Part model, mm, in its own coordinate system. Face numbers are marked on the shaded views. A direction names the side the tool comes from. Round coordinates to 2 decimals unless told otherwise and drop trailing zeros. Order: outer loops, then holes, each group sorted by start corner. A loop starts at its lowest first (then second) coordinate and runs counter-clockwise, first axis right, second up. Notation, with made-up numbers: (49, 65.5) - (106, 65.5) arc R20 cw to (106, 75.5) - close; hole circle Ø2 at (-6, 43.5). An arc over 180 degrees is marked (long way). Answer as a JSON object with one key per item and string values.
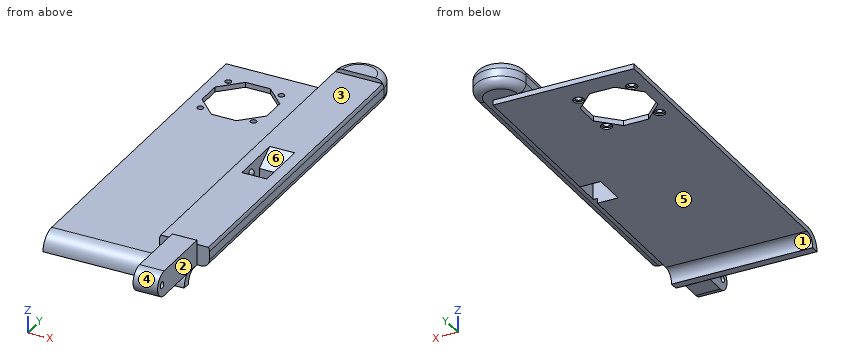
```python
from build123d import *

# Parameters (mm, degrees)
BOSS_EXTRUDE1_DEPTH = 7.5
FILLET1_R           = 5
SKETCH2_W           = 15
SKETCH2_H           = 20
CUT_EXTRUDE1_DEPTH  = 152.492574075
FILLET6_R           = 5
CUT_EXTRUDE2_DEPTH  = 152.848641746
BOSS_EXTRUDE2_DEPTH = 80
BOSS_EXTRUDE3_START = 5
BOSS_EXTRUDE3_DEPTH = 5
SKETCH12_W          = 12.5
SKETCH12_H          = 20
CUT_EXTRUDE3_DEPTH  = 3
SKETCH13_W          = 2.5
SKETCH13_H          = 200
CUT_EXTRUDE4_DEPTH  = 160.863222787
SKETCH14_R          = 1.85
CUT_EXTRUDE5_DEPTH  = 10
SKETCH15_R          = 3.25
CUT_EXTRUDE6_DEPTH  = 1
CUT_EXTRUDE7_DEPTH  = 7.5


with BuildPart() as part:
    # Sketch1 → Boss-Extrude1 (new, symmetric)
    with BuildSketch(Plane.XY):
        with BuildLine():
            Line((-15, 100), (-15, -100))
            Line((-15, -100), (-7.4, -100))
            Line((-7.4, -100), (-7.4, -150))
            Line((-7.4, -150), (7.4, -150))
            Line((7.4, -150), (7.4, -100))
            Line((7.4, -100), (15, -100))
            Line((15, -100), (15, 100))
            ThreePointArc((15, 100), (0, 115), (-15, 100))
        make_face()
    extrude(amount=BOSS_EXTRUDE1_DEPTH, both=True)

    # Fillet1
    fillet1_edges = [part.edges().sort_by_distance(p)[0] for p in [
        (-15, 0, -7.5),
        (0, 115, -7.5),
        (15, 0, 7.5),
        (0, 115, 7.5),
        (15, 0, -7.5),
        (-15, 0, 7.5),
    ]]
    fillet(fillet1_edges, radius=FILLET1_R)

    # Sketch2 → Cut-Extrude1 (cut, through all)
    with BuildSketch(Plane.XY.offset(7.5)):
        with Locations((0, -10)):
            Rectangle(SKETCH2_W, SKETCH2_H)
    extrude(amount=-CUT_EXTRUDE1_DEPTH, mode=Mode.SUBTRACT)

    # Sketch5 → Cut-Revolve1 (revolve, cut)
    with BuildSketch(Plane.XY):
        with BuildLine():
            Line((-7.4, -140), (-5.4, -140))
            ThreePointArc((-5.4, -140), (-5.985786438, -138.585786438), (-7.4, -138))
            Line((-7.4, -138), (-7.4, -140))
        make_face()
        with BuildLine():
            Line((7.4, -140), (5.4, -140))
            ThreePointArc((5.4, -140), (5.985786438, -138.585786438), (7.4, -138))
            Line((7.4, -138), (7.4, -140))
        make_face()
    revolve(axis=Axis((-35.580304025, -140, 0), (1, 0, 0)), mode=Mode.SUBTRACT)

    # Fillet6
    fillet6_edges = [part.edges().sort_by_distance(p)[0] for p in [
        (7.4, -150, 0),
        (-7.4, -150, 0),
    ]]
    fillet(fillet6_edges, radius=FILLET6_R)

    # Sketch7 → Cut-Extrude2 (cut, through all)
    with BuildSketch(Plane(origin=(7.4, 0, 0), x_dir=(0, 0, -1), z_dir=(1, 0, 0))):
        with BuildLine():
            Line((-7.5, -137.5), (-7.5, -150))
            Line((-7.5, -150), (7.5, -150))
            Line((7.5, -150), (7.5, -137.5))
            ThreePointArc((7.5, -137.5), (0, -145), (-7.5, -137.5))
        make_face()
    extrude(amount=-CUT_EXTRUDE2_DEPTH, mode=Mode.SUBTRACT)

    # Sketch9 → Revolve2 (revolve)
    with BuildSketch(Plane.XY):
        with BuildLine():
            Line((-7.5, -10), (-5.5, -10))
            ThreePointArc((-5.5, -10), (-6.085786438, -8.585786438), (-7.5, -8))
            Line((-7.5, -8), (-7.5, -10))
        make_face()
        with BuildLine():
            Line((7.5, -10), (5.5, -10))
            ThreePointArc((5.5, -10), (6.085786438, -8.585786438), (7.5, -8))
            Line((7.5, -8), (7.5, -10))
        make_face()
    revolve(axis=Axis((-32.251262552, -10, 0), (1, 0, 0)))

    # Sketch10 → Boss-Extrude2 (add)
    with BuildSketch(Plane(origin=(0, 0, 0), x_dir=(0, 0, -1), z_dir=(1, 0, 0))):
        with BuildLine():
            Line((7.5, -100), (7.5, 100))
            Line((7.5, 100), (10.5, 100))
            Line((10.5, 100), (10.5, -98.519259302))
            ThreePointArc((10.5, -98.519259302), (12.584119567, -103.288955309), (17.5, -105))
            Line((17.5, -105), (17.5, -110))
            ThreePointArc((17.5, -110), (10.428932188, -107.071067812), (7.5, -100))
        make_face()
    extrude(amount=-BOSS_EXTRUDE2_DEPTH)

    # Sketch11 → Boss-Extrude3 (add)
    with BuildSketch(Plane(origin=(0, 0, 0), x_dir=(0, 0, -1), z_dir=(1, 0, 0)).offset(BOSS_EXTRUDE3_START)):
        with BuildLine():
            Line((17.5, -110), (17.5, -105))
            ThreePointArc((17.5, -105), (12.584119567, -103.288955309), (10.5, -98.519259302))
            Line((10.5, -98.519259302), (10.5, 100))
            Line((10.5, 100), (7.5, 100))
            Line((7.5, 100), (7.5, -100))
            ThreePointArc((7.5, -100), (10.428932188, -107.071067812), (17.5, -110))
        make_face()
    extrude(amount=-BOSS_EXTRUDE3_DEPTH)

    # Sketch12 → Cut-Extrude3 (cut)
    with BuildSketch(Plane(origin=(0, 0, -10.5), x_dir=(-1, 0, 0), z_dir=(0, 0, -1))):
        with Locations((1.25, -10)):
            Rectangle(SKETCH12_W, SKETCH12_H)
    extrude(amount=-CUT_EXTRUDE3_DEPTH, mode=Mode.SUBTRACT)

    # Sketch13 → Cut-Extrude4 (cut, through all)
    with BuildSketch(Plane.ZY.offset(15)):
        with Locations((6.25, 0)):
            Rectangle(SKETCH13_W, SKETCH13_H)
    extrude(amount=-CUT_EXTRUDE4_DEPTH, mode=Mode.SUBTRACT)

    # Sketch14 → Cut-Extrude5 (cut)
    with BuildSketch(Plane(origin=(0, 0, -10.5), x_dir=(-1, 0, 0), z_dir=(0, 0, -1))):
        with Locations(Location((70, 51.480740698, 0), (0, 0, 90))):
            Circle(SKETCH14_R)
        with Locations(Location((70, 83.480740698, 0), (0, 0, 90))):
            Circle(SKETCH14_R)
        with Locations(Location((38, 83.480740698, 0), (0, 0, 90))):
            Circle(SKETCH14_R)
        with Locations(Location((38, 51.480740698, 0), (0, 0, 90))):
            Circle(SKETCH14_R)
        Polygon((61.5, 86.980740698), (46.5, 86.980740698), (34.5, 74.980740698), (34.5, 59.980740698), (46.5, 47.980740698), (61.5, 47.980740698), (73.5, 59.980740698), (73.5, 74.980740698), align=None)
    extrude(amount=-CUT_EXTRUDE5_DEPTH, mode=Mode.SUBTRACT)

    # Sketch15 → Cut-Extrude6 (cut)
    with BuildSketch(Plane(origin=(0, 0, -10.5), x_dir=(-1, 0, 0), z_dir=(0, 0, -1))):
        with Locations(Location((70, 83.480740698, 0), (0, 0, 90))):
            Circle(SKETCH15_R)
        with Locations(Location((38, 83.480740698, 0), (0, 0, 90))):
            Circle(SKETCH15_R)
        with Locations(Location((38, 51.480740698, 0), (0, 0, 90))):
            Circle(SKETCH15_R)
        with Locations(Location((70, 51.480740698, 0), (0, 0, 90))):
            Circle(SKETCH15_R)
    extrude(amount=-CUT_EXTRUDE6_DEPTH, mode=Mode.SUBTRACT)

    # Sketch16 → Cut-Extrude7 (cut, symmetric)
    with BuildSketch(Plane(origin=(0, 0, 0), x_dir=(0, 0, -1), z_dir=(1, 0, 0))):
        Polygon((2.5, 0), (-5, 12), (-5, 0), align=None)
    extrude(amount=CUT_EXTRUDE7_DEPTH, both=True, mode=Mode.SUBTRACT)


solid = part.part
```
Item 1: Tool access for the marked faces 4, 5 and 6: list every direction of +Z, -Z, +X, -X, +Y, -Y with a clear straight run to the whole face (end or side of a thin tool).
Taken from the geometry:
{"face 4": "+X, -X, -Y", "face 5": "-Z, +X, -X, +Y", "face 6": "+Z"}
Item 2: Drop flat-ended pins along their axis: P1, Ø6, axis at x = -38, y = 83.48, coming from the -Z side; P2, Ø3.5, axis at x = -50.5, z = -9.5, coming from the +Y side; P3, Ø1.5, axis at y = 33.5, z = -9.5, coming from the +X side. Give the stop position or say it passes through.
Taken from the geometry:
{"P1": "z = -9.5", "P2": "y = 100", "P3": "x = 5"}
Item 3: Cut at C-C (x = -27). Write the cut outline in (y, z), plus the area to 3 significant figures.
Taken from the geometry:
{"outline": "(-110, -17.5) - (-105, -17.5) arc R6.5 cw to (-98.52, -10.5) - (100, -10.5) - (100, -7.5) - (-100, -7.5) arc R10 ccw to start", "area": "652 mm2"}
Item 4: Cut at D-D (z = -14.75). Write the cut outline in (x, y).
Taken from the geometry:
{"outline": "(-80, -109.61) - (5, -109.61) - (5, -104.62) - (-80, -104.62) - close"}
Item 5: Cut at B-B (y = -85.5). Write the cut outline in (x, z), plus the area to 3 significant figures.
Taken from the geometry:
{"outline": "(-80, -10.5) - (5, -10.5) - (5, -7.5) - (10, -7.5) arc R5 ccw to (15, -2.5) - (15, 2.5) arc R5 ccw to (14.33, 5) - (-14.33, 5) arc R5 ccw to (-15, 2.5) - (-15, -2.5) arc R5 ccw to (-10, -7.5) - (-80, -7.5) - close", "area": "618 mm2"}
Item 6: Two-plate mould, pull along Y, no slides. Class the marked faces 1, 2 and 3: pulls with the +Y half, pulls with the -Y half, needs draft (parallel to the pull), parting line crosses it, or undercut.
Taken from the geometry:
{"face 1": "pulls with the +Y half", "face 2": "needs draft", "face 3": "undercut"}
Item 7: Cut at A-A (x = 0). Write the cut outline in (y, z), plus the area to 3 significant figures.
Taken from the geometry:
{"outline": "(-137.5, -7.5) - (-100, -7.5) arc R10 ccw to (-110, -17.5) - (-105, -17.5) arc R6.5 cw to (-98.52, -10.5) - (-20, -10.5) - (-20, 5) - (-100, 5) - (-100, 7.5) - (-137.5, 7.5) arc R7.5 ccw to start; (0, -10.5) - (100, -10.5) - (100, -7.5) - (110, -7.5) arc R5 ccw to (115, -2.5) - (115, 2.5) arc R5 ccw to (110, 7.5) - (100, 7.5) - (100, 5) - (12, 5) - (0, -2.5) - close", "area": "3,660 mm2"}
Item 8: Probe L1, parallel to X at y = 66, z = -10; L2, parallel to X at y = 6, z = 2.25; L3, parallel to Z at x = -70, y = -68. List the from-to ranges inside material, lowest first. Write a range as from..to.
Taken from the geometry:
{"L1": "-80..-73.5, -34.5..5", "L2": "-15..-7.5, 7.5..15", "L3": "-10.5..-7.5"}
